from build123d import *

# Parameters (mm, degrees)
BOSS_EXTRUDE1_DEPTH = 250
CUT_EXTRUDE1_REACH  = 45
SKETCH2_W           = 10.8
SKETCH2_H           = 114
SKETCH3_W           = 248
SKETCH3_H           = 35
SKETCH3_W_2         = 247.6
SKETCH3_H_2         = 34.6
CUT_EXTRUDE2_DEPTH  = 0.2
FILLET1_R           = 0.5
SKETCH4_R           = 14
CUT_EXTRUDE3_DEPTH  = 14.8


with BuildPart() as part:
    # Sketch1 → Boss-Extrude1 (new body)
    with BuildSketch(Plane.XY):
        Polygon((0, 3), (9.091796068, 3), (10.8, 3.854101966), (10.8, 37.323614418), (6.450873429, 40), (0, 40), (0, 43), (7.3, 43), (13.8, 39), (13.8, 2), (9.8, 0), (0, 0), align=None)
    extrude(amount=BOSS_EXTRUDE1_DEPTH)

    # Sketch2 → Cut-Extrude1 (cut, up to next)
    with BuildSketch(Plane.XZ, mode=Mode.PRIVATE) as cut_extrude1_sk1:
        with Locations((5.4, 125)):
            Rectangle(SKETCH2_W, SKETCH2_H)
    cut_extrude1_tool1 = extrude(cut_extrude1_sk1.sketch, amount=-CUT_EXTRUDE1_REACH, mode=Mode.PRIVATE) & part.part
    add(cut_extrude1_tool1.solids().sort_by_distance((5.4, 0, 125))[0], mode=Mode.SUBTRACT)

    # Sketch3 → Cut-Extrude2 (cut)
    with BuildSketch(Plane(origin=(13.8, 0, 0), x_dir=(0, 0, -1), z_dir=(1, 0, 0))):
        with Locations((-125, 20.5)):
            Rectangle(SKETCH3_W, SKETCH3_H)
        with Locations((-125, 20.5)):
            Rectangle(SKETCH3_W_2, SKETCH3_H_2, mode=Mode.SUBTRACT)
    extrude(amount=-CUT_EXTRUDE2_DEPTH, mode=Mode.SUBTRACT)

    # Fillet1
    fillet1_edges = [part.edges().sort_by_distance(p)[0] for p in [
        (13.8, 39, 125),
        (13.8, 2, 125),
        (9.8, 0, 216),
        (7.3, 43, 125),
        (9.8, 0, 34),
    ]]
    fillet(fillet1_edges, radius=FILLET1_R)

    # Sketch4 → Cut-Extrude3 (cut, through all)
    with BuildSketch(Plane(origin=(13.8, 0, 0), x_dir=(0, 0, -1), z_dir=(1, 0, 0))):
        with Locations((-220, 20.514809699)):
            Circle(SKETCH4_R)
    extrude(amount=-CUT_EXTRUDE3_DEPTH, mode=Mode.SUBTRACT)


solid = part.part
Build history of the part. All positions in model axes, mm. A direction names the side the tool comes from. Round coordinates to 2 decimals unless told otherwise and drop trailing zeros. Write each loop counter-clockwise with the first axis right and the second up, starting at its lowest first coordinate (ties: lowest second). Pieces come first, ordered by that corner, then holes. Notation, with made-up numbers: M 73,66.5 L 91,66.5 A26 ccw 91,102.5 Z; hole C -2,56.5 d1. An arc over 180 degrees is marked long. Use CSV: the item, a comma, the result in double quotes.
1. Tool access for faces 1 (the face through (5, 1, 68)), 2 (the face through (8.66, 38.64, 123.25)), 3 (the face through (10.45, 41.06, 123.25)): list every direction of +Z, -Z, +X, -X, +Y, -Y with a clear straight run to the whole face (end or side of a thin tool).
Reply:
face 1,"-X, -Y"
face 2,"+Z, -Z, -X"
face 3,"+Z, -Z, +X, +Y"
2. Saw through at A-A (z = 220). Give the cut face in (x, y).
Reply:
outline,"M 0,0 L 9.68,0 A0.5 ccw 9.91,0.05 L 13.52,1.86 A0.5 ccw 13.8,2.31 L 13.8,3 L 13.6,3 L 13.6,3.2 L 13.8,3.2 L 13.8,6.51 L 10.8,6.51 L 10.8,3.85 L 9.09,3 L 0,3 Z; M 0,40 L 6.45,40 L 10.8,37.32 L 10.8,34.51 L 13.8,34.51 L 13.8,37.8 L 13.6,37.8 L 13.6,38 L 13.8,38 L 13.8,38.72 A0.5 ccw 13.56,39.15 L 7.42,42.93 A0.5 ccw 7.16,43 L 0,43 Z"
3. Wall check: probe 1 along Y at (x, z) = (6, 20); probe 2 along X at (y, z) = (30.5, 111); probe 3 along Z at (x, y) = (12.75, 20.5). Give the ranges that are in metal, low to high. Write a range as from..to.
Reply:
probe 1,"y = 0..3, 40..43"
probe 2,"x = 10.8..13.8"
probe 3,"z = 0..206, 234..250"
4. Flat gauge pins, fed straight in: pin 1 (11 mm diameter, centred on y = 22.5, z = 168.5, fed in from -X); pin 2 (6 mm diameter, centred on x = 11.5, z = 66, fed in from +Y). Where does each tip first touch, or does it go through?
Reply:
pin 1,"stops at x = 10.8"
pin 2,"stops at y = 42.26"
5. Saw through at C-C (z = 90.5). Give the cut face in (x, y), plus the area to 3 significant figures.
Reply:
outline,"M 0,40 L 6.45,40 L 10.8,37.32 L 10.8,0.5 L 13.52,1.86 A0.5 ccw 13.8,2.31 L 13.8,3 L 13.6,3 L 13.6,3.2 L 13.8,3.2 L 13.8,37.8 L 13.6,37.8 L 13.6,38 L 13.8,38 L 13.8,38.72 A0.5 ccw 13.56,39.15 L 7.42,42.93 A0.5 ccw 7.16,43 L 0,43 Z"
area,"150 mm²"
6. Saw through at D-D (y = 14.5). Give the cut face in (x, z).
Reply:
outline,"M 10.8,0 L 13.8,0 L 13.8,1 L 13.6,1 L 13.6,1.2 L 13.8,1.2 L 13.8,207.36 L 10.8,207.36 Z; M 10.8,232.64 L 13.8,232.64 L 13.8,248.8 L 13.6,248.8 L 13.6,249 L 13.8,249 L 13.8,250 L 10.8,250 Z"
7. Saw through at B-B (y = 27). Give the cut face in (x, z).
Reply:
outline,"M 10.8,0 L 13.8,0 L 13.8,1 L 13.6,1 L 13.6,1.2 L 13.8,1.2 L 13.8,207.59 L 10.8,207.59 Z; M 10.8,232.41 L 13.8,232.41 L 13.8,248.8 L 13.6,248.8 L 13.6,249 L 13.8,249 L 13.8,250 L 10.8,250 Z"
